The figure shows three views and two pictorial views of one solid part (mm, origin at its lowest corner). Answer the questions. A direction names the side the tool comes from. Round coordinates to 2 decimals unless told otherwise and drop trailing zeros. Write each loop counter-clockwise with the first axis right and the second up, starting at its lowest first coordinate (ties: lowest second). Pieces come first, ordered by that corner, then holes.
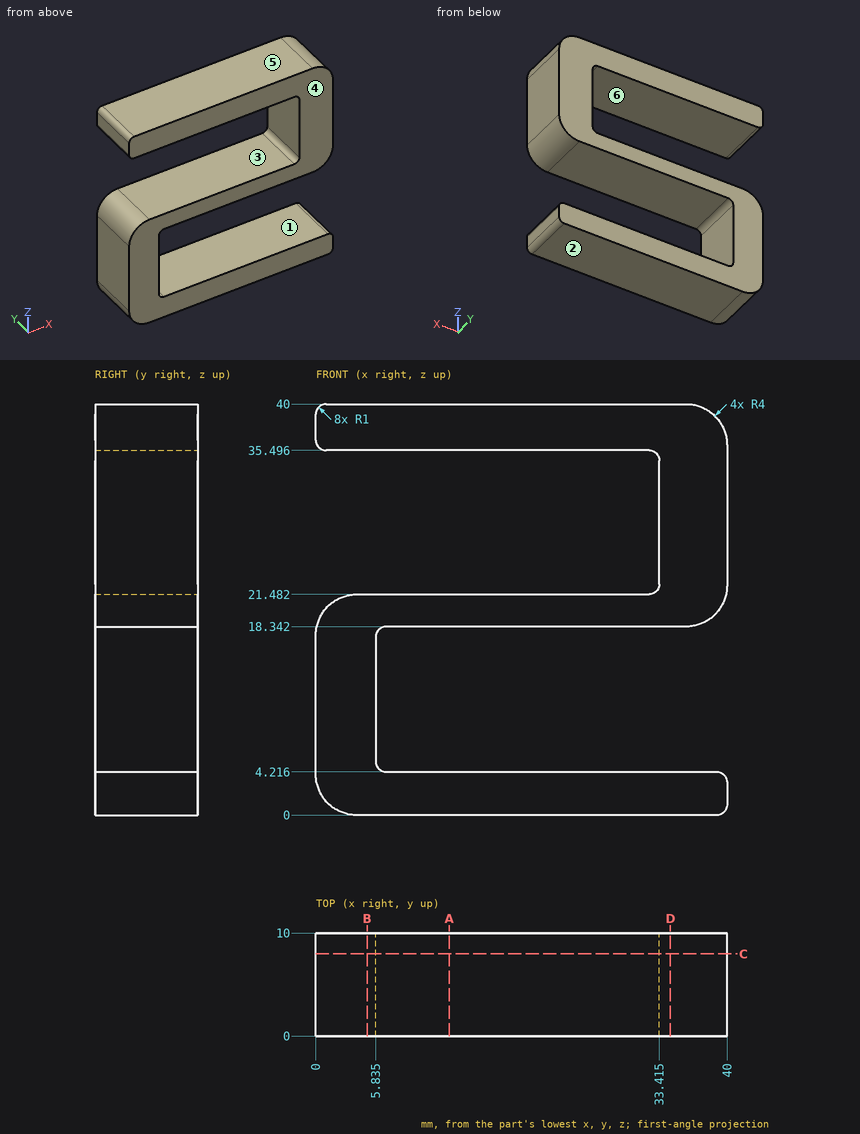
Q1. Which of the six approach directions +Z, -Z, +X, -X, +Y, -Y give full straight-line access (tool end or side, diameter ignored) to the marked faces 1, 2 and 3?
Verdict:
face 1: +X, +Y, -Y
face 2: -Z, +X, -X, +Y, -Y
face 3: -X, +Y, -Y
Q2. Section C-C (y = 8) is taken. Determine the outline of the cut face in (x, z) (1 decimal).
Verdict:
outline: (0, 4) arc R4 ccw to (4, 0) - (39, 0) arc R1 ccw to (40, 1) - (40, 3.2) arc R1 ccw to (39, 4.2) - (6.8, 4.2) arc R1 cw to (5.8, 5.2) - (5.8, 17.3) arc R1 cw to (6.8, 18.3) - (36, 18.3) arc R4 ccw to (40, 22.3) - (40, 36) arc R4 ccw to (36, 40) - (1, 40) arc R1 ccw to (0, 39) - (0, 36.5) arc R1 ccw to (1, 35.5) - (32.4, 35.5) arc R1 cw to (33.4, 34.5) - (33.4, 22.5) arc R1 cw to (32.4, 21.5) - (4, 21.5) arc R4 ccw to (0, 17.5) - close
Q3. Determine the mould class of the marked faces 4, 5 and 6 for opening direction Z: pulls with the +Z half, pulls with the -Z half, needs draft (parallel to the pull), parting line crosses it, or undercut.
Verdict:
face 4: needs draft
face 5: pulls with the +Z half
face 6: undercut
Q4. Section B-B (x = 5) is taken. Determine the outline of the cut face in (y, z) (1 decimal), then the cut area to 3 significant figures.
Verdict:
outline: (0, 0) - (10, 0) - (10, 21.5) - (0, 21.5) - close; (0, 35.5) - (10, 35.5) - (10, 40) - (0, 40) - close
area: 260 mm2
Q5. Flat-ended cylindrical pins translate along their axes: pin 1 Ø5 at (y, z) = (7, 11) entering from +X (1 decimal); pin 2 Ø5 at (y, z) = (7, 29.5) entering from -X (1 decimal). Find the tip coordinate at first contact, or state that the pin passes through.
Verdict:
pin 1: stops at x = 5.8
pin 2: stops at x = 33.4
Q6. Section D-D (x = 34.5) is taken. Determine the outline of the cut face in (y, z) (1 decimal), then the cut area to 3 significant figures.
Verdict:
outline: (0, 0) - (10, 0) - (10, 4.2) - (0, 4.2) - close; (0, 18.3) - (10, 18.3) - (10, 40) - (0, 40) - close
area: 259 mm2
Q7. Straight lines are drawn through the part: probe 1 along Z at (x, y) = (19, 5) (1 decimal); probe 2 along X at (y, z) = (4.5, 30) (1 decimal); probe 3 along X at (y, z) = (6, 11) (1 decimal). For each, find the intervals that lie inside material, in ascending order.
Verdict:
probe 1: z = 0 to 4.2, 18.3 to 21.5, 35.5 to 40
probe 2: x = 33.4 to 40
probe 3: x = 0 to 5.8
Q8. Section A-A (x = 13) is taken. Determine the outline of the cut face in (y, z) (1 decimal), then the cut area to 3 significant figures.
Verdict:
outline: (0, 0) - (10, 0) - (10, 4.2) - (0, 4.2) - close; (0, 18.3) - (10, 18.3) - (10, 21.5) - (0, 21.5) - close; (0, 35.5) - (10, 35.5) - (10, 40) - (0, 40) - close
area: 119 mm2
